```python
from build123d import *

# Parameters (mm, degrees)
SKETCH1_W           = 100
SKETCH1_H           = 80
SKETCH1_R           = 26
BOSS_EXTRUDE1_DEPTH = 70
SKETCH2_R           = 32.5
CUT_EXTRUDE1_DEPTH  = 27
BOSS_EXTRUDE2_START = 1
SKETCH4_R           = 32.5
SKETCH4_R_2         = 30.25
BOSS_EXTRUDE2_DEPTH = 1
SKETCH5_R           = 35
CUT_EXTRUDE2_DEPTH  = 19
CUT_EXTRUDE3_START  = -7
SKETCH6_R           = 32.5
CUT_EXTRUDE3_DEPTH  = 7


with BuildPart() as part:
    # Sketch1 → Boss-Extrude1 (new body)
    with BuildSketch(Plane(origin=(0, 0, 0), x_dir=(1, 0, 0), z_dir=(0, 1, 0))):
        Rectangle(SKETCH1_W, SKETCH1_H)
        with Locations(Location((0, 0, 0), (0, 0, 270))):
            Circle(SKETCH1_R, mode=Mode.SUBTRACT)
    extrude(amount=BOSS_EXTRUDE1_DEPTH)

    # Sketch2 → Cut-Extrude1 (cut)
    with BuildSketch(Plane(origin=(0, 70, 0), x_dir=(1, 0, 0), z_dir=(0, 1, 0))):
        with Locations(Location((0, 0, 0), (0, 0, 270))):
            Circle(SKETCH2_R)
    extrude(amount=-CUT_EXTRUDE1_DEPTH, mode=Mode.SUBTRACT)

    # Sketch4 → Boss-Extrude2 (add)
    with BuildSketch(Plane(origin=(0, 43, 0), x_dir=(1, 0, 0), z_dir=(0, 1, 0)).offset(BOSS_EXTRUDE2_START)):
        with Locations(Location((0, 0, 0), (0, 0, 270))):
            Circle(SKETCH4_R)
        with Locations(Location((0, 0, 0), (0, 0, 270))):
            Circle(SKETCH4_R_2, mode=Mode.SUBTRACT)
    extrude(amount=-BOSS_EXTRUDE2_DEPTH)

    # Sketch5 → Cut-Extrude2 (cut)
    with BuildSketch(Plane(origin=(0, 70, 0), x_dir=(1, 0, 0), z_dir=(0, 1, 0))):
        with Locations(Location((0, 0, 0), (0, 0, 270))):
            Circle(SKETCH5_R)
    extrude(amount=-CUT_EXTRUDE2_DEPTH, mode=Mode.SUBTRACT)

    # Sketch6 → Cut-Extrude3 (cut)
    with BuildSketch(Plane.XZ.offset(CUT_EXTRUDE3_START)):
        with Locations(Location((0, 0, 0), (0, 0, 90))):
            Circle(SKETCH6_R)
    extrude(amount=CUT_EXTRUDE3_DEPTH, mode=Mode.SUBTRACT)


solid = part.part
```
Verification items for the finished model (mm, model axes). A direction names the side the tool comes from. Coordinates: 2 decimals unless noted, no trailing zeros. Write each loop counter-clockwise with the first axis right and the second up, starting at its lowest first coordinate (ties: lowest second). Pieces come first, ordered by that corner, then holes. Notation, with made-up numbers: M 42.5,15.25 L 76.5,15.25 A26 cw 76.5,50.25 Z; hole C -9,74.25 d2. An arc over 180 degrees is marked long. One line per item, written item: value.
Item 1: Section check B-B, the plane z = 8. Record the boundary of the cut face in (x, y).
Check sheet entries:
outline: M -50,0 L -31.5,0 L -31.5,7 L -24.74,7 L -24.74,43 L -29.17,43 L -29.17,44 L -31.5,44 L -31.5,51 L -34.07,51 L -34.07,70 L -50,70 Z; M 24.74,7 L 31.5,7 L 31.5,0 L 50,0 L 50,70 L 34.07,70 L 34.07,51 L 31.5,51 L 31.5,44 L 29.17,44 L 29.17,43 L 24.74,43 Z
Item 2: Section check D-D, the plane y = 56.5. Record the boundary of the cut face in (x, z), plus the area to 3 significant figures.
Check sheet entries:
outline: M -50,-40 L 50,-40 L 50,40 L -50,40 Z; hole C 0,0 d70
area: 4,150 mm^2
Item 3: Access from +Z, -Z, +X, -X, +Y, -Y to the whole of each face (thin tool, end or side, straight path). Record for faces 4 (the cylindrical face through (-15.821, 24.748, -20.633)), 5 (the flat face through (23, 43, 13)), 6 (the flat face through (-22, 7, -15)).
Check sheet entries:
face 4: +Y, -Y
face 5: +Y
face 6: -Y
Item 4: Scan lines: line 1 along X through (y, z) = (58.75, 0); line 2 along Z through (x, y) = (-13, 52); line 3 along X through (y, z) = (37, 18.5). Record each from-to range of solid material in increasing order.
Check sheet entries:
line 1: x = -50 to -35, 35 to 50
line 2: z = -40 to -32.5, 32.5 to 40
line 3: x = -50 to -18.27, 18.27 to 50
Item 5: Mould release check, pull along Z, two halves, no side actions. Record for faces 1 (the cylindrical face through (-21, 61, -28)), 2 (the flat face through (-1, 35, 40)), 3 (the flat face through (50, 35, 1)): pulls with the +Z half, pulls with the -Z half, needs draft (parallel to the pull), parting line crosses it, or undercut.
Check sheet entries:
face 1: undercut
face 2: pulls with the +Z half
face 3: needs draft
Item 6: Section check C-C, the plane y = 36. Record the boundary of the cut face in (x, z).
Check sheet entries:
outline: M -50,-40 L 50,-40 L 50,40 L -50,40 Z; hole C 0,0 d52
Item 7: Section check A-A, the plane x = 0. Record the boundary of the cut face in (y, z).
Check sheet entries:
outline: M 0,-40 L 70,-40 L 70,-35 L 51,-35 L 51,-32.5 L 44,-32.5 L 44,-30.25 L 43,-30.25 L 43,-26 L 7,-26 L 7,-32.5 L 0,-32.5 Z; M 0,32.5 L 7,32.5 L 7,26 L 43,26 L 43,30.25 L 44,30.25 L 44,32.5 L 51,32.5 L 51,35 L 70,35 L 70,40 L 0,40 Z
